```python
from build123d import *

# Parameters (mm, degrees)
BOSS_EXTRUDE1_DEPTH                             = 170
SKETCH3_R                                       = 2
BOSS_EXTRUDE2_DEPTH                             = 5
SKETCH4_W                                       = 47.5
SKETCH4_H                                       = 4
BOSS_EXTRUDE3_DEPTH                             = 20
FILLET1_R                                       = 5
FILLET2_R                                       = 5
CSK_FOR_M3_FLAT_HEAD_MACHINE_SCREW1_D           = 3.2
CSK_FOR_M3_FLAT_HEAD_MACHINE_SCREW1_CSINK_D     = 6.3
CSK_FOR_M3_FLAT_HEAD_MACHINE_SCREW1_CSINK_ANGLE = 90
FILLET1_OF_MIRROR1_R                            = 5
FILLET2_OF_MIRROR1_R                            = 5


with BuildPart() as part:
    # Sketch1 → Boss-Extrude1 (new body)
    with BuildSketch(Plane(origin=(0, 0, 0), x_dir=(1, 0, 0), z_dir=(0, 1, 0))):
        with BuildLine():
            Line((-38.75, -50.75), (28.75, -50.75))
            ThreePointArc((28.75, -50.75), (35.821067812, -47.821067812), (38.75, -40.75))
            Line((38.75, -40.75), (38.75, 40.75))
            ThreePointArc((38.75, 40.75), (35.821067812, 47.821067812), (28.75, 50.75))
            Line((28.75, 50.75), (-38.75, 50.75))
            Line((-38.75, 50.75), (-38.75, -50.75))
        make_face()
        with BuildLine():
            Line((-36.75, 48.75), (26.75, 48.75))
            ThreePointArc((26.75, 48.75), (33.821067812, 45.821067812), (36.75, 38.75))
            Line((36.75, 38.75), (36.75, -38.75))
            ThreePointArc((36.75, -38.75), (33.821067812, -45.821067812), (26.75, -48.75))
            Line((26.75, -48.75), (-36.75, -48.75))
            Line((-36.75, -48.75), (-36.75, 48.75))
        make_face(mode=Mode.SUBTRACT)
    extrude(amount=BOSS_EXTRUDE1_DEPTH)

    # Sketch3 → Boss-Extrude2 (add)
    with BuildSketch(Plane(origin=(0, 170, 0), x_dir=(1, 0, 0), z_dir=(0, 1, 0))):
        with BuildLine():
            Line((-38.75, 50.75), (28.75, 50.75))
            ThreePointArc((28.75, 50.75), (35.821067812, 47.821067812), (38.75, 40.75))
            Line((38.75, 40.75), (38.75, -40.75))
            ThreePointArc((38.75, -40.75), (35.821067812, -47.821067812), (28.75, -50.75))
            Line((28.75, -50.75), (-38.75, -50.75))
            Line((-38.75, -50.75), (-38.75, 50.75))
        make_face()
        with Locations(Location((-31.75, -43.75, 0), (0, 0, 270))):
            Circle(SKETCH3_R, mode=Mode.SUBTRACT)
        with Locations(Location((-31.75, 43.75, 0), (0, 0, 270))):
            Circle(SKETCH3_R, mode=Mode.SUBTRACT)
        with Locations(Location((31.75, 43.75, 0), (0, 0, 270))):
            Circle(SKETCH3_R, mode=Mode.SUBTRACT)
        with Locations(Location((31.75, -43.75, 0), (0, 0, 270))):
            Circle(SKETCH3_R, mode=Mode.SUBTRACT)
        with BuildLine():
            Line((-36.75, 38.75), (-36.75, -38.75))
            Line((-36.75, -38.75), (-29.75, -38.75))
            ThreePointArc((-29.75, -38.75), (-27.628679656, -39.628679656), (-26.75, -41.75))
            Line((-26.75, -41.75), (-26.75, -48.75))
            Line((-26.75, -48.75), (26.75, -48.75))
            Line((26.75, -48.75), (26.75, -41.75))
            ThreePointArc((26.75, -41.75), (27.628679656, -39.628679656), (29.75, -38.75))
            Line((29.75, -38.75), (36.75, -38.75))
            Line((36.75, -38.75), (36.75, 38.75))
            Line((36.75, 38.75), (29.75, 38.75))
            ThreePointArc((29.75, 38.75), (27.628679656, 39.628679656), (26.75, 41.75))
            Line((26.75, 41.75), (26.75, 48.75))
            Line((26.75, 48.75), (-26.75, 48.75))
            Line((-26.75, 48.75), (-26.75, 41.75))
            ThreePointArc((-26.75, 41.75), (-27.628679656, 39.628679656), (-29.75, 38.75))
            Line((-29.75, 38.75), (-36.75, 38.75))
        make_face(mode=Mode.SUBTRACT)
    extrude(amount=BOSS_EXTRUDE2_DEPTH)

    # Sketch4 → Boss-Extrude3 (add)
    with BuildSketch(Plane(origin=(0, 10, 0), x_dir=(-1, 0, 0), z_dir=(0, -1, 0))):
        with Locations((5, -52.75)):
            Rectangle(SKETCH4_W, SKETCH4_H)
    boss_extrude3 = extrude(amount=BOSS_EXTRUDE3_DEPTH)

    # Fillet1
    fillet1_edges = [part.edges().sort_by_distance(p)[0] for p in [
        (18.75, -10, 52.75),
        (-28.75, -10, 52.75),
    ]]
    fillet(fillet1_edges, radius=FILLET1_R)

    # Fillet2
    # the kernel refuses this fillet: 5 mm, written as the material it takes off along each edge
    with BuildSketch(Plane(origin=(-40.997448714, 10, 54.75), x_dir=(0, -1, 0), z_dir=(1, 0, 0))) as fillet2_piece_1:
        with BuildLine():
            CenterArc((4.898979486, 5), FILLET2_R, 191.536959033, 78.463040967)
            Line((0, 4), (-0.09797959, 3.98))
            ThreePointArc((-0.09797959, 3.98), (-0.1, 2), (-0.1, 0))
            Line((-0.1, 0), (0, -0.1))
            Line((0, -0.1), (4.898979486, -0.1))
            Line((4.898979486, -0.1), (4.898979486, 0))
        make_face()
    extrude(amount=71.994897428, mode=Mode.SUBTRACT)

    # CSK for M3 Flat Head Machine Screw1 (through all)
    with Locations(Plane.XY.offset(54.75)):
        with Locations((13.75, -5), (-23.75, -5)):
            csk_for_m3_flat_head_machine_screw1 = CounterSinkHole(CSK_FOR_M3_FLAT_HEAD_MACHINE_SCREW1_D / 2, CSK_FOR_M3_FLAT_HEAD_MACHINE_SCREW1_CSINK_D / 2, counter_sink_angle=CSK_FOR_M3_FLAT_HEAD_MACHINE_SCREW1_CSINK_ANGLE)

    # Mirror1: Boss-Extrude3, CSK for M3 Flat Head Machine Screw1 across plane
    add(boss_extrude3.mirror(Plane.XY))
    add(csk_for_m3_flat_head_machine_screw1.mirror(Plane.XY), mode=Mode.SUBTRACT)

    # Fillet1 of Mirror1
    fillet1_of_mirror1_edges = [part.edges().sort_by_distance(p)[0] for p in [
        (18.75, -10, -52.75),
        (-28.75, -10, -52.75),
    ]]
    fillet(fillet1_of_mirror1_edges, radius=FILLET1_OF_MIRROR1_R)

    # Fillet2 of Mirror1
    # the kernel refuses this fillet: 5 mm, written as the material it takes off along each edge
    with BuildSketch(Plane(origin=(-40.997448714, 10, -54.75), x_dir=(0, -1, 0), z_dir=(1, 0, 0))) as fillet2_of_mirror1_piece_1:
        with BuildLine():
            CenterArc((4.898979486, -5), FILLET2_OF_MIRROR1_R, 90, 78.463040967)
            Line((0, -4), (-0.09797959, -3.98))
            ThreePointArc((-0.09797959, -3.98), (-0.1, -2), (-0.1, 0))
            Line((-0.1, 0), (0, 0.1))
            Line((0, 0.1), (4.898979486, 0.1))
            Line((4.898979486, 0.1), (4.898979486, 0))
        make_face()
    extrude(amount=71.994897428, mode=Mode.SUBTRACT)


solid = part.part
```
Check sheet for the modelled part. Datum: model origin and axes. Units: mm. A direction names the side the tool comes from. Coordinates: 2 decimals unless noted, no trailing zeros. Loops run counter-clockwise (first coordinate to the right, second up) from the corner with the lowest first, then second, coordinate; pieces in that order, holes last.
1) Sectioned sample at C-C (x = 21). Record the boundary of the cut face in (y, z), and give its area (3 significant figures).
2) Material ranges on probe 1 along Z at (x, y) = (-9, 34); probe 2 along X at (y, z) = (173, 43); probe 3 along X at (y, z) = (135.5, 24.5), recorded low to high.
3) Gauge pin test, flat ends, axial feed: pin 1 (11 mm diameter, centred on x = -34, z = -43, fed in from -Y); pin 2 (20 mm diameter, centred on x = 1.5, y = 44, fed in from -Z); pin 3 (2.5 mm diameter, centred on x = 13.75, y = -5, fed in from +Z); pin 4 (10 mm diameter, centred on x = 2.5, y = 31, fed in from +Z). Record the tip position at first contact, or that the pin passes through.
4) Sectioned sample at B-B (x = -31.75). Record the boundary of the cut face in (y, z), and give its area (3 significant figures).
5) Release check for a two-part mould opening along Z. For faces 4 (the face through (-5, -2, 54.75)), 5 (the face through (-5, -5, -50.75)), 6 (the face through (38.75, 86, -1)) record: released by +Z, released by -Z, zero draft, split by the parting line, or undercut.
6) Sectioned sample at D-D (y = 159). Record the boundary of the cut face in (x, z).
7) Sectioned sample at A-A (z = 29). Record the boundary of the cut face in (x, y), and give its area (3 significant figures).
8) Access from +Z, -Z, +X, -X, +Y, -Y to the whole of each face (thin tool, end or side, straight path). Record for faces 1 (the face through (-28.75, 3, -53)), 2 (the face through (-26.75, 172, -45)), 3 (the face through (-36.75, 86, -1)).
Check sheet entries:
1. outline: (0, -50.75) - (175, -50.75) - (175, -48.75) - (0, -48.75) - close; (0, 48.75) - (175, 48.75) - (175, 50.75) - (0, 50.75) - close
1. area: 700 mm2
2. probe 1: z = -50.75 to -48.75, 48.75 to 50.75
2. probe 2: x = -38.75 to -33.6, -29.9 to -26.75, 26.75 to 29.9, 33.6 to 38.49
2. probe 3: x = -38.75 to -36.75, 36.75 to 38.75
3. pin 1: stops at y = 0
3. pin 2: stops at z = -50.75
3. pin 3: passes through
3. pin 4: stops at z = 50.75
4. outline: (0, -50.75) - (175, -50.75) - (175, -45.75) - (170, -45.75) - (170, -48.75) - (0, -48.75) - close; (0, 48.75) - (170, 48.75) - (170, 45.75) - (175, 45.75) - (175, 50.75) - (0, 50.75) - close; (170, -41.75) - (175, -41.75) - (175, -38.75) - (170, -38.75) - close; (170, 38.75) - (175, 38.75) - (175, 41.75) - (170, 41.75) - close
4. area: 760 mm2
5. face 4: released by +Z
5. face 5: undercut
5. face 6: zero draft
6. outline: (-38.75, -50.75) - (28.75, -50.75) arc R10 ccw to (38.75, -40.75) - (38.75, 40.75) arc R10 ccw to (28.75, 50.75) - (-38.75, 50.75) - close; hole (-36.75, -48.75) - (26.75, -48.75) arc R10 ccw to (36.75, -38.75) - (36.75, 38.75) arc R10 ccw to (26.75, 48.75) - (-36.75, 48.75) - close
7. outline: (-38.75, 0) - (-36.75, 0) - (-36.75, 175) - (-38.75, 175) - close; (36.75, 0) - (38.75, 0) - (38.75, 175) - (36.75, 175) - close
7. area: 700 mm2
8. face 1: -Z, -X, +Y, -Y
8. face 2: +Y, -Y
8. face 3: -Y
